For this review, take the finished solid that the model builds, in its own axes (mm). Coordinates: 2 decimals unless noted, no trailing zeros. Loops run counter-clockwise (first coordinate to the right, second up) from the corner with the lowest first, then second, coordinate; pieces in that order, holes last. Notation, with made-up numbers: (49.5, 70.25) - (103.5, 70.25) arc R21 cw to (103.5, 84.25) - close; hole circle Ø2 at (42.5, 11.5). An arc over 180 degrees is marked (long way). Answer as a JSON object with one key per item and string values. Group by question number.
Item 1: To check wall thickness, follow line 1 (Z direction, x = -57.15, y = 2.3); line 2 (X direction, y = 2.35, z = 5); line 3 (X direction, y = 1.5, z = 36.5). State the ranges of each line that lie inside material, in increasing order.
Item 2: We need section B-B (z = 6). Give the boundary of the cut face in (x, y) (3 decimals), then the cut area to 3 significant figures.
Item 3: We need section C-C (y = 1.45). State how many separate pieces and enclosed holes the cut face has, then the cut area to 3 significant figures.
Item 4: Clearance check with flat-ended pins moving along their axes: pin 1 (6 mm diameter, centred on x = 0, z = 7.1, fed in from +Y) (1 decimal); pin 2 (10 mm diameter, centred on x = -40.5, z = 11.5, fed in from -Y); pin 3 (1.6 mm diameter, centred on y = 1, z = 17, fed in from -X); pin 4 (1 mm diameter, centred on x = -31.5, y = 2, fed in from +Z). State where each tip first meets the part, or that it passes through.
Item 5: We need section A-A (x = -65). Give the boundary of the cut face in (y, z) (3 decimals).
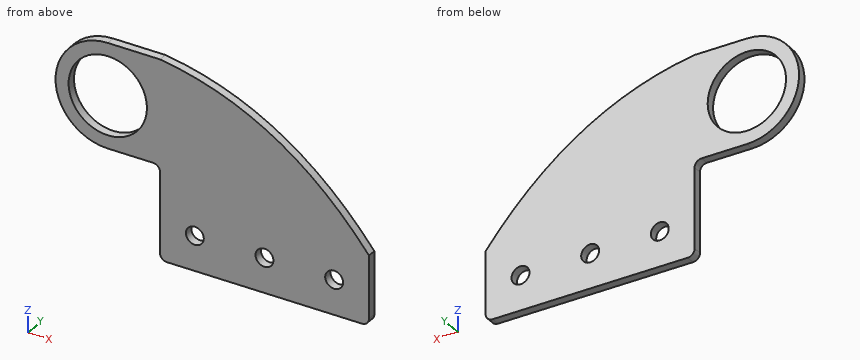
from build123d import *

# Parameters (mm, degrees)
SKETCH1_R           = 14.2875
SKETCH1_R_2         = 3.2639
BOSS_EXTRUDE1_DEPTH = 3.175
FILLET1_R           = 2.54


with BuildPart() as part:
    # Sketch1 → Boss-Extrude1 (new body)
    with BuildSketch(Plane(origin=(0, 0, 0), x_dir=(1, 0, 0), z_dir=(0, 1, 0))):
        with BuildLine():
            Line((-38.1, -28.693802537), (-57.15, -28.693802537))
            ThreePointArc((-57.15, -28.693802537), (-76.2, -47.743802537), (-57.15, -66.793802537))
            Line((-57.15, -66.793802537), (-38.1, -66.793802537))
            add(Edge.make_bspline(
                [(38.1, -19.803802537), (6.35, -60.443802537), (-38.1, -66.793802537)],
                knots=[0, 0, 0, 1, 1, 1], degree=2))
            Line((38.1, -19.803802537), (38.1, 5.596197463))
            Line((38.1, 5.596197463), (-38.1, 5.596197463))
            Line((-38.1, 5.596197463), (-38.1, -28.693802537))
        make_face()
        with Locations((-57.15, -47.743802537)):
            Circle(SKETCH1_R, mode=Mode.SUBTRACT)
        with Locations((-25.4, -7.103802537)):
            Circle(SKETCH1_R_2, mode=Mode.SUBTRACT)
        with Locations((0, -7.103802537)):
            Circle(SKETCH1_R_2, mode=Mode.SUBTRACT)
        with Locations((25.4, -7.103802537)):
            Circle(SKETCH1_R_2, mode=Mode.SUBTRACT)
    extrude(amount=BOSS_EXTRUDE1_DEPTH)

    # Fillet1
    fillet1_edges = [part.edges().sort_by_distance(p)[0] for p in [
        (-38.1, 1.5875, 28.693802537),
        (-38.1, 1.5875, -5.596197463),
        (38.1, 1.5875, -5.596197463),
    ]]
    fillet(fillet1_edges, radius=FILLET1_R)


solid = part.part
Check sheet entries:
{
 "1": {"line 1": "z = 28.69 to 33.46, 62.03 to 66.79", "line 2": "x = -38.1 to -27.9, -22.9 to -2.5, 2.5 to 22.9, 27.9 to 38.1", "line 3": "x = -72.53 to -65.97, -48.33 to 23.02"},
 "2": {"outline": "(-38.1, 0) - (-28.472, 0) - (-28.472, 3.175) - (-38.1, 3.175) - close; (-22.328, 0) - (-3.072, 0) - (-3.072, 3.175) - (-22.328, 3.175) - close; (3.072, 0) - (22.328, 0) - (22.328, 3.175) - (3.072, 3.175) - close; (28.472, 0) - (38.1, 0) - (38.1, 3.175) - (28.472, 3.175) - close", "area": "183 mm2"},
 "3": {"separate pieces": "1", "enclosed holes": "4", "area": "4,810 mm2"},
 "4": {"pin 1": "passes through", "pin 2": "stops at y = 0", "pin 3": "stops at x = -38.1", "pin 4": "stops at z = 65.75"},
 "5": {"outline": "(0, 30.386) - (3.175, 30.386) - (3.175, 35.806) - (0, 35.806) - close; (0, 59.682) - (3.175, 59.682) - (3.175, 65.101) - (0, 65.101) - close"}
}
